Part model, mm, in its own coordinate system. Face numbers are marked on the shaded views. A direction names the side the tool comes from. Coordinates: 2 decimals unless noted, no trailing zeros. Loops run counter-clockwise (first coordinate to the right, second up) from the corner with the lowest first, then second, coordinate; pieces in that order, holes last. Notation, with made-up numbers: M 61,20 L 84,20 A24 cw 84,45 Z; hole C -26,-29.75 d2. An arc over 180 degrees is marked long. Answer as a JSON object with one key per item and string values. Group by question number.
1. Saw through at C-C on y = -6.5. Write the cut outline in (x, z).
2. Saw through at B-B on x = 2.25. Count the separate pieces of the cut face and the enclosed holes in it, then the cut area to 3 significant figures.
3. Saw through at A-A on x = 8.5. Write the cut outline in (y, z).
4. Saw through at D-D on x = 15.5. Write the cut outline in (y, z), then the cut area to 3 significant figures.
5. 3-axis set-ups, long thin cutter, end or side, ignore diameter. For the marked faces 5, 6, 7 and 8: which of +Z, -Z, +X, -X, +Y, -Y reach the whole face in a straight line?
6. Drill centre lines: L1, parallel to Y at x = 6.5, z = 16; L2, parallel to Y at x = 4, z = -16; L3, parallel to X at y = 9, z = -20. Where is each one in solid material? Low to high.
7. Mould opens along Z. For the marked faces 1, 2, 3 and 4 say: released by +Z, released by -Z, zero draft, split by the parting line, or undercut.
8. Drop flat-ended pins along their axis: pin 1 Ø3.5 at (x, y) = (17, -5.5) entering from -Z; pin 2 Ø8 at (x, z) = (16.5, -15) entering from -Y; pin 3 Ø5.5 at (x, y) = (3, -18) entering from -Z; pin 4 Ø2 at (y, z) = (-11.5, -8) entering from +X. Give the stop position or say it passes through.
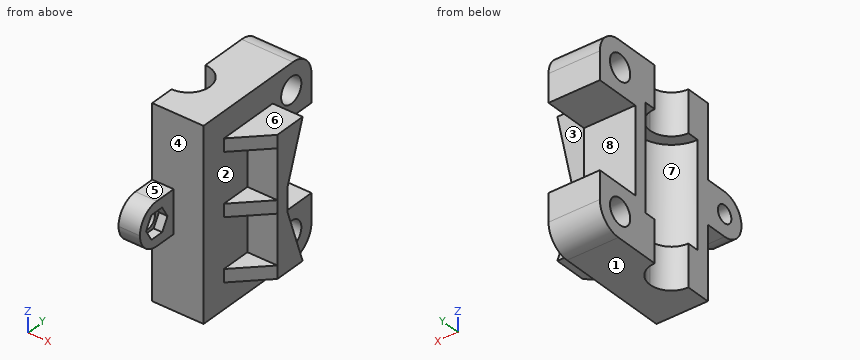
from build123d import *

# Parameters (mm, degrees)
SKETCH1_W               = 44
SKETCH1_H               = 32
BOSS_EXTRUDE1_DEPTH     = 12
SKETCH2_W               = 24.5
SKETCH2_H               = 15.5
CUT_EXTRUDE1_DEPTH      = 7.75
FILLET1_R               = 7.75
CUT_EXTRUDE2_DEPTH      = 40.661851949
CUT_EXTRUDE2_DEPTH_BACK = 40.661851949
SKETCH4_R               = 3
SKETCH4_W               = 20
SKETCH4_H               = 10.5
CUT_EXTRUDE3_DEPTH      = 30.732137495
SKETCH5_W               = 5.5
SKETCH5_H               = 3
BOSS_EXTRUDE4_DEPTH     = 7
CHAMFER1_SIZE           = 7
SKETCH6_W               = 11.5
SKETCH6_H               = 7
CUT_EXTRUDE5_DEPTH      = 30.732137495
FILLET4_R               = 5.5
SKETCH7_W               = 10
SKETCH7_H               = 10
SKETCH7_R               = 2
BOSS_EXTRUDE5_DEPTH     = 5
CUT_EXTRUDE6_START      = -2
SKETCH8_R               = 2
CUT_EXTRUDE6_DEPTH      = 2
FILLET5_R               = 5


with BuildPart() as part:
    # Sketch1 → Boss-Extrude1 (new body)
    with BuildSketch(Plane(origin=(0, 0, 0), x_dir=(0, 0, -1), z_dir=(1, 0, 0))):
        Rectangle(SKETCH1_W, SKETCH1_H)
    extrude(amount=BOSS_EXTRUDE1_DEPTH)

    # Sketch2 → Cut-Extrude1 (cut)
    with BuildSketch(Plane(origin=(0, 0, 0), x_dir=(0, 0, -1), z_dir=(1, 0, 0))):
        with Locations((0, -5.25)):
            Rectangle(SKETCH2_W, SKETCH2_H)
    extrude(amount=CUT_EXTRUDE1_DEPTH, mode=Mode.SUBTRACT)

    # Fillet1
    fillet1_edges = [part.edges().sort_by_distance(p)[0] for p in [
        (7.75, 2.5, 0),
        (7.75, -13, 0),
    ]]
    fillet(fillet1_edges, radius=FILLET1_R - 0.0001)  # a hair under: the kernel refuses the full size

    # Sketch3 → Cut-Extrude2 (cut, two sides: drawn at the far end of the back side and taken through both)
    with BuildSketch(Plane.XY.offset(-12.25).offset(-CUT_EXTRUDE2_DEPTH_BACK)):
        with BuildLine():
            ThreePointArc((0, -10.25), (3.535533906, -8.785533906), (5, -5.25))
            ThreePointArc((5, -5.25), (3.535533906, -1.714466094), (0, -0.25))
            Line((0, -0.25), (0, -10.25))
        make_face()
        with BuildLine():
            Line((0, -10.25), (0, -0.25))
            ThreePointArc((0, -0.25), (-5, -5.25), (0, -10.25))
        make_face()
    extrude(amount=CUT_EXTRUDE2_DEPTH + CUT_EXTRUDE2_DEPTH_BACK, mode=Mode.SUBTRACT)

    # Sketch4 → Cut-Extrude3 (cut, through all)
    with BuildSketch(Plane(origin=(12, 0, 0), x_dir=(0, 0, -1), z_dir=(1, 0, 0))):
        with Locations((-16, 10)):
            Circle(SKETCH4_R)
        with Locations((16, 10)):
            Circle(SKETCH4_R)
        with Locations((0, 10.75)):
            Rectangle(SKETCH4_W, SKETCH4_H)
    extrude(amount=-CUT_EXTRUDE3_DEPTH, mode=Mode.SUBTRACT)

    # Sketch5 → Boss-Extrude4 (add)
    with BuildSketch(Plane(origin=(12, 0, 0), x_dir=(0, 0, -1), z_dir=(1, 0, 0))):
        Polygon((-16, -3), (-16, 4.5), (-2.75, -3), align=None)
        Polygon((-2.75, -3), (-16, 4.5), (-2.75, 0), align=None)
        with Locations((0, -1.5)):
            Rectangle(SKETCH5_W, SKETCH5_H)
        Polygon((2.75, -3), (2.75, 0), (16, 4.5), align=None)
        Polygon((16, -3), (2.75, -3), (16, 4.5), align=None)
    extrude(amount=BOSS_EXTRUDE4_DEPTH)

    # Chamfer1
    chamfer1_edges = [part.edges().sort_by_distance(p)[0] for p in [
        (12, -3, 0),
    ]]
    chamfer(chamfer1_edges, length=CHAMFER1_SIZE - 0.0001)  # a hair under: the kernel refuses the full size

    # Sketch6 → Cut-Extrude5 (cut, through all)
    with BuildSketch(Plane(origin=(12, 0, 0), x_dir=(0, 0, -1), z_dir=(1, 0, 0))):
        with Locations((-7.25, -6.5)):
            Rectangle(SKETCH6_W, SKETCH6_H)
        with Locations((7.25, -6.5)):
            Rectangle(SKETCH6_W, SKETCH6_H)
    extrude(amount=CUT_EXTRUDE5_DEPTH, mode=Mode.SUBTRACT)

    # Fillet4
    fillet4_edges = [part.edges().sort_by_distance(p)[0] for p in [
        (6, 16, 22),
        (6, 16, -22),
    ]]
    fillet(fillet4_edges, radius=FILLET4_R)

    # Sketch7 → Boss-Extrude5 (add)
    with BuildSketch(Plane(origin=(0, 0, 0), x_dir=(0, 0, -1), z_dir=(1, 0, 0))):
        with Locations((0, -21)):
            Rectangle(SKETCH7_W, SKETCH7_H)
        with Locations((0, -21)):
            Circle(SKETCH7_R, mode=Mode.SUBTRACT)
    extrude(amount=BOSS_EXTRUDE5_DEPTH)

    # Sketch8 → Cut-Extrude6 (cut)
    with BuildSketch(Plane(origin=(5, 0, 0), x_dir=(0, 0, -1), z_dir=(1, 0, 0)).offset(CUT_EXTRUDE6_START)):
        Polygon((0, -24.175426481), (2.75, -22.58771324), (2.75, -19.41228676), (0, -17.824573519), (-2.75, -19.41228676), (-2.75, -22.58771324), align=None)
        with Locations((0, -21)):
            Circle(SKETCH8_R, mode=Mode.SUBTRACT)
    extrude(amount=CUT_EXTRUDE6_DEPTH, mode=Mode.SUBTRACT)

    # Fillet5
    fillet5_edges = [part.edges().sort_by_distance(p)[0] for p in [
        (2.5, -26, -5),
        (2.5, -26, 5),
    ]]
    fillet(fillet5_edges, radius=FILLET5_R - 0.0001)  # a hair under: the kernel refuses the full size


solid = part.part
Outcome:
{
 "1": {"outline": "M 4.84,-22 L 12,-22 L 12,-16 L 15.5,-16 L 15.5,-13 L 12,-13 L 12,-1.5 L 15.5,-1.5 L 15.5,1.5 L 12,1.5 L 12,13 L 15.5,13 L 15.5,16 L 12,16 L 12,22 L 4.84,22 L 4.84,12.25 L 7.65,12.25 L 7.65,-12.25 L 4.84,-12.25 Z"},
 "2": {"separate pieces": "2", "enclosed holes": "3", "area": "668 mm²"},
 "3": {"outline": "M -16,-22 L 10.5,-22 A5.5 ccw 16,-16.5 L 16,-10 L 5.5,-10 L 5.5,10 L 16,10 L 16,16.5 A5.5 ccw 10.5,22 L -16,22 Z; hole C 10,-16 d6; hole C 10,16 d6"},
 "4": {"outline": "M -6.5,-16 L 4.5,-16 L 0,-2.75 L 0,2.75 L 4.5,16 L -6.5,16 L -6.5,13 L -3,13 L -3,1.5 L -6.5,1.5 L -6.5,-1.5 L -3,-1.5 L -3,-13 L -6.5,-13 Z", "area": "187 mm²"},
 "5": {"face 5": "+Z, +X, -X, -Y", "face 6": "+Z, +X, +Y, -Y", "face 7": "-X", "face 8": "+X, -X, +Y"},
 "6": {"L1": "y = -16 to 7, 13 to 16", "L2": "y = -16 to -8.25, -2.25 to 7, 13 to 16", "L3": "x = 0 to 12"},
 "7": {"face 1": "released by -Z", "face 2": "undercut", "face 3": "undercut", "face 4": "zero draft"},
 "8": {"pin 1": "stops at z = -16", "pin 2": "stops at y = -9.5", "pin 3": "stops at z = -22", "pin 4": "stops at x = 12"}
}
